For this review, take the finished solid that the model builds, in its own axes (mm). A direction names the side the tool comes from. Coordinates: 2 decimals unless noted, no trailing zeros. Write each loop counter-clockwise with the first axis right and the second up, starting at its lowest first coordinate (ties: lowest second). Pieces come first, ordered by that corner, then holes. Notation, with made-up numbers: (51, 35) - (96, 35) arc R15 ccw to (96, 62) - close; hole circle Ø5 at (14, -8.75). An arc over 180 degrees is marked (long way). Use one line per item in the form item = value. Start each with the question number.
1) Mouldability with a two-part tool opening along X and no side actions: class faces 3 (the flat face through (116, 45.5, 0)), 4 (the flat face through (-128, -37, 0)), 5 (the flat face through (165, 0, 0)) as pulls with the +X half, pulls with the -X half, needs draft (parallel to the pull), parting line crosses it, or undercut.
2) We need section C-C (y = -37.5). Count the separate pieces of the cut face and the enclosed holes in it, plus the area to 3 significant figures.
3) Insertion check: P1, Ø5.5, axis at x = 137.5, y = 15, coming from the -Z side; P2, Ø7.5, axis at x = -27.5, y = -15, coming from the -Z side; P3, Ø0.9, axis at y = 40.5, z = -1.5, coming from the +X side. Each pin has a flat end and moves straight along its axis. Give the tip position at first contact, or say it passes through.
4) We need section B-B (x = 110). Give the boundary of the cut face in (y, z).
5) Tool access review of faces 1 (the cylindrical face through (140.744, -14.28, 0.17)), 2 (the cylindrical face through (-0.242, 43.245, 2.958)): name each direction out of +Z, -Z, +X, -X, +Y, -Y from which nothing blocks a thin tool from reaching the whole face with its end or side.
6) We need section A-A (x = 66). Give the boundary of the cut face in (y, z), plus the area to 3 significant figures.
7) For L1, parallel to Y at x = -82.5, z = 2.25; L2, parallel to Y at x = -66, z = -2.55; L3, parallel to X at y = 0, z = 0.5, list the stretches that pass through material, from the lowest coordinate up. Write a range as from..to.
Autodesk Inventor part; units mm, degrees
ref_plane "YZ Plane" through (0, 0, 0) normal (1, 0, 0) x (0, 1, 0)
ref_plane "XZ Plane" through (0, 0, 0) normal (0, 1, 0) x (-1, 0, 0)
ref_plane "XY Plane" through (0, 0, 0) normal (0, 0, 1) x (1, 0, 0)
sketch "Sketch5" plane through (0, 0, 0) normal (0, 0, 1) x (1, 0, 0)
  line L0 (-165, 45.5) -> (165, 45.5)
  line L1 (165, 45.5) -> (165, -45.5)
  line L2 (165, -45.5) -> (-165, -45.5)
  line L3 (-165, -45.5) -> (-165, 45.5)
  point P0 (0, 0)
  point P1 (0, 45.5)
  point P2 (165, 0)
  dimension "d8" = 330
  dimension "d9" = 91
extrude "Extrusion5" add sketch "Sketch5" along normal mid plane 12
sketch "Sketch6" plane through (0, 0, 6) normal (0, 0, 1) x (1, 0, 0)
  circle A0 centre (132, -37.5) radius 3
  circle A1 centre (66, -37.5) radius 3
  circle A2 centre (-66, -37.5) radius 3
  circle A3 centre (-132, -37.5) radius 3
  circle A4 centre (0, -37.5) radius 3
  circle A5 centre (132, 37.75) radius 3
  circle A6 centre (66, 37.75) radius 3
  circle A7 centre (-66, 37.75) radius 3
  circle A8 centre (-132, 37.75) radius 3
  circle A9 centre (0, 37.75) radius 3
  line L0 (165, 45.5) -> (-165, 45.5)
  circle A10 centre (132, -37.5) radius 5
  point P0 (-165, -45.5)
  point P1 (0, 0)
  dimension "d12" = 66
  dimension "d13" = 66
  dimension "d14" = 66
  dimension "d17" = 6
  dimension "d20" = 66
  dimension "d22" = 66
  dimension "d23" = 66
  dimension "d24" = 66
  dimension "d25" = 6
  dimension "d26" = 66
  dimension "d27" = 75.25
  dimension "d64" = 7.75
  dimension "d65" = 91
  dimension "d103" = 10
hole "Hole1" at (-132, 37.75, 6) at (132, 37.75, 6) at (66, 37.75, 6) at (0, 37.75, 6) at (-66, 37.75, 6) at (132, -37.5, 6) at (66, -37.5, 6) at (0, -37.5, 6) at (-66, -37.5, 6) at (-132, -37.5, 6) direction (0, 0, -1) diameter 7 end through all counterbore diameter 11 counterbore depth 6
sketch "Sketch7" plane through (0, 0, 6) normal (0, 0, 1) x (1, 0, 0)
  line L0 (-165, 45.5) -> (-165, -45.5)
  line L1 (-165, -45.5) -> (165, -45.5)
  line L2 (165, -45.5) -> (165, 45.5)
  circle A0 centre (137.5, -15) radius 4
  circle A1 centre (137.5, 15) radius 4
  circle A2 centre (82.5, -15) radius 4
  circle A3 centre (82.5, 15) radius 4
  circle A4 centre (27.5, -15) radius 4
  circle A5 centre (27.5, 15) radius 4
  circle A6 centre (-27.5, -15) radius 4
  circle A7 centre (-27.5, 15) radius 4
  circle A8 centre (-82.5, -15) radius 4
  circle A9 centre (-82.5, 15) radius 4
  circle A10 centre (-137.5, -15) radius 4
  circle A11 centre (-137.5, 15) radius 4
  point P0 (0, 0)
  dimension "d35" = 27.5
  dimension "d36" = 30
  dimension "d37" = 15
  dimension "d38" = 8
  dimension "d41" = 55
  dimension "d46" = 27.5
hole "Hole2" at (137.5, -15, 6) at (137.5, 15, 6) at (82.5, 15, 6) at (82.5, -15, 6) at (27.5, -15, 6) at (27.5, 15, 6) at (-27.5, 15, 6) at (-27.5, -15, 6) at (-82.5, -15, 6) at (-82.5, 15, 6) at (-137.5, 15, 6) at (-137.5, -15, 6) direction (0, 0, -1) diameter 6.647 end through all
sketch "Sketch8" plane through (-165, -45.5, 6) normal (-1, 0, 0) x (0, 0, 1)
  line L0 (-12, 0) -> (-12, 91)
  line L1 (-11.5, 14.5) -> (-12, 14.5)
  line L2 (-12, 14.5) -> (-12, 76.5)
  line L3 (-12, 76.5) -> (-11.5, 76.5)
  line L4 (-11.5, 76.5) -> (-11.5, 14.5)
  point P0 (-6, 45.5)
  point P1 (-11.5, 45.5)
  dimension "d54" = 0.5
  dimension "d55" = 62
extrude "Extrusion6" cut sketch "Sketch8" against normal through all
sketch "Sketch9" plane through (0, 0, 6) normal (0, 0, 1) x (1, 0, 0)
  circle A0 centre (66, 37.75) radius 3.5
  line L0 (165, 45.5) -> (-165, 45.5)
  line L1 (82.5, 30.5) -> (82.5, 60.5) construction
  line L2 (91.5, 30.5) -> (91.5, 60.5)
  line L3 (73.5, 60.5) -> (73.5, 30.5)
  arc A1 (73.5, 30.5) -> (91.5, 30.5) centre (82.5, 30.5) ccw
  arc A2 (91.5, 60.5) -> (73.5, 60.5) centre (82.5, 60.5) ccw
  line L4 (0, 0) -> (0, 10.6364) construction
  line L5 (0, 0) -> (-13.5916, 0) construction
  line L6 (-82.5, 30.5) -> (-82.5, 60.5) construction
  line L7 (-91.5, 30.5) -> (-91.5, 60.5)
  line L8 (-73.5, 60.5) -> (-73.5, 30.5)
  arc A3 (-91.5, 30.5) -> (-73.5, 30.5) centre (-82.5, 30.5) ccw
  arc A4 (-73.5, 60.5) -> (-91.5, 60.5) centre (-82.5, 60.5) ccw
  circle A5 centre (-137.5, 15) radius 3.3235
  circle A6 centre (-82.5, -15) radius 3.3235
  circle A7 centre (-27.5, 15) radius 3.3235
  circle A8 centre (27.5, -15) radius 3.3235
  circle A9 centre (82.5, 15) radius 3.3235
  circle A10 centre (137.5, -15) radius 3.3235
  circle A11 centre (137.5, 15) radius 3.3235
  circle A12 centre (82.5, -15) radius 3.3235
  circle A13 centre (27.5, 15) radius 3.3235
  circle A14 centre (-27.5, -15) radius 3.3235
  circle A15 centre (-82.5, 15) radius 3.3235
  circle A16 centre (-137.5, -15) radius 3.3235
  circle A17 centre (-66, -37.5) radius 5.5
  circle A18 centre (66, -37.5) radius 5.5
  circle A19 centre (-66, 37.75) radius 5.5
  circle A20 centre (66, 37.75) radius 5.5
  circle A21 centre (-132, 37.75) radius 5.5
  circle A22 centre (132, 37.75) radius 5.5
  circle A23 centre (0, 37.75) radius 5.5
  circle A24 centre (132, -37.5) radius 5.5
  circle A25 centre (0, -37.5) radius 5.5
  circle A26 centre (-132, -37.5) radius 5.5
  line L9 (165, 45.5) -> (-165, 45.5)
  line L10 (-165, 45.5) -> (-165, -45.5)
  line L11 (-165, -45.5) -> (165, -45.5)
  line L12 (165, -45.5) -> (165, 45.5)
  point P0 (82.5, 45.5)
  point P1 (-82.5, 45.5)
  dimension "d58" = 16.5
  dimension "d59" = 30
  dimension "d61" = 18
extrude "Extrusion7" cut sketch "Sketch9" against normal through all contours L2 A1 L3 L0 | L0 L3 A2 L2 | L8 A3 L7 L0 | L0 L7 A4 L8
sketch "Sketch10" plane through (0, 0, 6) normal (0, 0, 1) x (1, 0, 0)
  line L0 (-165, -45.5) -> (165, -45.5)
  line L1 (165, -45.5) -> (165, 45.5)
  circle A0 centre (110, 0) radius 5
  circle A1 centre (55, 0) radius 5
  circle A2 centre (0, 0) radius 5
  circle A3 centre (-55, 0) radius 5
  circle A4 centre (-110, 0) radius 5
  dimension "d66" = 55
  dimension "d70" = 55
  dimension "d75" = 10
hole "Hole3" at (110, 0, 6) at (55, 0, 6) at (0, 0, 6) at (-55, 0, 6) at (-110, 0, 6) direction (0, 0, -1) diameter 10 end through all
sketch "Sketch11" plane through (165, -31, -5.5) normal (1, 0, 0) x (0, 0, -1)
  circle A0 centre (-5.5, 11) radius 3
  circle A1 centre (-5.5, 51) radius 3
  point P0 (-5.5, 31)
  dimension "d86" = 40
  dimension "d87" = 20
  dimension "d88" = 6
hole "Hole4" at (165, -20, 0) at (165, 20, 0) direction (-1, 0, 0) diameter 4.134 depth 15 tip angle 118
sketch "Sketch12" plane through (-165, -31, -5.5) normal (-1, 0, 0) x (0, 0, 1)
  circle A0 centre (5.5, 11) radius 2.067
  circle A1 centre (5.5, 51) radius 2.067
  circle A2 centre (5.5, 11) radius 2.067
  circle A3 centre (5.5, 51) radius 2.067
  point P0 (5.5, 31)
hole "Hole5" at (-165, -20, 0) at (-165, 20, 0) direction (1, 0, 0) diameter 4.134 depth 15 tip angle 118
chamfer "Chamfer2" distance 15 angle 45 2 edges at (165, -45.5, 0) (-165, -45.5, 0)
sketch "Sketch13" plane through (0, 0, 6) normal (0, 0, 1) x (1, 0, 0)
  circle A0 centre (0, 37.75) radius 5.5
  line L0 (165, 45.5) -> (145, 45.5)
  line L1 (145, 45.5) -> (145, 30.5)
  line L2 (145, 30.5) -> (165, 30.5)
  line L3 (165, 30.5) -> (165, 45.5)
  line L4 (0, 37.75) -> (0, 63.3817) construction
  line L5 (-165, 45.5) -> (-145, 45.5)
  line L6 (-145, 45.5) -> (-145, 30.5)
  line L7 (-145, 30.5) -> (-165, 30.5)
  line L8 (-165, 30.5) -> (-165, 45.5)
  dimension "d107" = 15
  dimension "d108" = 20
extrude "Extrusion8" cut sketch "Sketch13" against normal through all contours L3 L2 L1 L0 | L5 L6 L7 L8
fillet "Fillet1" radius 9 2 edges at (145, 30.5, 0.25) (-145, 30.5, 0.25)
chamfer "Chamfer3" distance 3 angle 45 2 edges at (145, 45.5, 0) (-145, 45.5, 0)
equation "\"d13\" = d12"
equation "\"d14\" = d12"
equation "\"d20\" = d12"
equation "\"d23\" = d22"
equation "\"d24\" = d22"
equation "\"d26\" = d22"
properties part number "BC-10017" material "Alumínio 7075"
Determined:
q1.face_3 = needs draft
q1.face_4 = undercut
q1.face_5 = pulls with the +X half
q2.separate_pieces = 6
q2.enclosed_holes = 0
q2.area = 3,250 mm²
q3.P1 = through
q3.P2 = -5.5
q3.P3 = 145
q4.outline = (-45.5, -6) - (-31, -6) - (-31, -5.5) - (-5, -5.5) - (-5, 6) - (-45.5, 6) - close; (5, -5.5) - (31, -5.5) - (31, -6) - (45.5, -6) - (45.5, 6) - (5, 6) - close
q5.face_1 = +Z, -Z
q5.face_2 = +Z
q6.outline = (-45.5, -6) - (-41, -6) - (-41, 0) - (-43, 0) - (-43, 6) - (-45.5, 6) - close; (-34, -6) - (-31, -6) - (-31, -5.5) - (31, -5.5) - (31, -6) - (34.25, -6) - (34.25, 0) - (32.25, 0) - (32.25, 6) - (-32, 6) - (-32, 0) - (-34, 0) - close; (41.25, -6) - (45.5, -6) - (45.5, 6) - (43.25, 6) - (43.25, 0) - (41.25, 0) - close
q6.area = 845 mm²
q7.L1 = -45.5..-18.32, -11.68..11.68, 18.32..21.5
q7.L2 = -45.5..-41, -34..34.25, 41.25..45.5
q7.L3 = -165..-115, -105..-60, -50..-5, 5..50, 60..105, 115..165
